Model file for the job. Use its own axes, mm. Face numbers are marked on the shaded views. A direction names the side the tool comes from. Round coordinates to 2 decimals unless told otherwise and drop trailing zeros. Loops run counter-clockwise (first coordinate to the right, second up) from the corner with the lowest first, then second, coordinate; pieces in that order, holes last. Notation, with made-up numbers: M -13,27.25 L 41,27.25 A33 cw 41,60.25 Z; hole C -31,49 d9. An arc over 180 degrees is marked long. Answer in a Markdown table with one row per item.
from build123d import *

# Parameters (mm, degrees)
F0_W     = 0.1
F0_H     = 20.0163984491
F0_W_2   = 0.2
F0_H_2   = 20
F0_W_3   = 0.3
F0_W_4   = 0.4
F0_W_5   = 0.5
F0_W_6   = 0.6
F0_W_7   = 0.7
F0_W_8   = 0.8
F0_W_9   = 0.9
F0_W_10  = 1
F0_R     = 0.05
F0_R_2   = 0.1
F0_R_3   = 0.15
F0_R_4   = 0.2
F0_R_5   = 0.25
F0_R_6   = 0.3
F0_R_7   = 0.35
F0_R_8   = 0.4
F0_R_9   = 0.45
F0_R_10  = 0.5
F1_DEPTH = 10
F2_W     = 1
F2_H     = 20
F2_W_2   = 0.2
F2_W_3   = 0.5
F2_W_4   = 0.9
F2_W_5   = 0.7
F2_W_6   = 0.8
F2_W_7   = 0.6
F2_R     = 0.35
F2_R_2   = 0.2
F2_R_3   = 0.15
F2_R_4   = 0.1
F2_W_8   = 0.3
F2_R_5   = 0.3
F2_R_6   = 0.4
F2_R_7   = 0.05
F2_R_8   = 0.45
F2_R_9   = 0.5
F2_R_10  = 0.25
F2_W_9   = 0.4
F2_W_10  = 0.1
F2_H_2   = 20.0163984491
F3_DEPTH = 50


with BuildPart() as f1:
    # F0 (on Top) → F1 (new body)
    with BuildSketch(Plane.XY):
        with BuildLine():
            Line((30, 29.7358127656), (-10, 29.7358127656))
            ThreePointArc((-10, 29.7358127656), (-24.1421356237, 23.8779483894), (-30, 9.7358127656))
            Line((-30, 9.7358127656), (-30, -22.3076807681))
            Line((-30, -22.3076807681), (10, -22.3076807681))
            ThreePointArc((10, -22.3076807681), (24.1421356237, -16.4498163918), (30, -2.3076807681))
            Line((30, -2.3076807681), (30, 29.7358127656))
        make_face()
        with Locations((-25.3179286689, -1.6637592667)):
            Rectangle(F0_W, F0_H, mode=Mode.SUBTRACT)
        with Locations((-20.1679286689, -1.6719584912)):
            Rectangle(F0_W_2, F0_H_2, mode=Mode.SUBTRACT)
        with Locations((-14.9179286689, -1.6719584912)):
            Rectangle(F0_W_3, F0_H_2, mode=Mode.SUBTRACT)
        with Locations((-9.5679286689, -1.6719584912)):
            Rectangle(F0_W_4, F0_H_2, mode=Mode.SUBTRACT)
        with Locations((-4.1179286689, -1.6719584912)):
            Rectangle(F0_W_5, F0_H_2, mode=Mode.SUBTRACT)
        with Locations((1.4320713311, -1.6719584912)):
            Rectangle(F0_W_6, F0_H_2, mode=Mode.SUBTRACT)
        with Locations((7.0820713311, -1.6719584912)):
            Rectangle(F0_W_7, F0_H_2, mode=Mode.SUBTRACT)
        with Locations((12.8320713311, -1.6719584912)):
            Rectangle(F0_W_8, F0_H_2, mode=Mode.SUBTRACT)
        with Locations((18.6820713311, -1.6719584912)):
            Rectangle(F0_W_9, F0_H_2, mode=Mode.SUBTRACT)
        with Locations((24.6320713311, -1.6719584912)):
            Rectangle(F0_W_10, F0_H_2, mode=Mode.SUBTRACT)
        with Locations((-25.3179286689, 13.3444399579)):
            Circle(F0_R, mode=Mode.SUBTRACT)
        with Locations((-20.1679286689, 13.3444399579)):
            Circle(F0_R_2, mode=Mode.SUBTRACT)
        with Locations((-14.9179286689, 13.3444399579)):
            Circle(F0_R_3, mode=Mode.SUBTRACT)
        with Locations((-9.5679286689, 13.3444399579)):
            Circle(F0_R_4, mode=Mode.SUBTRACT)
        with Locations((-4.1179286689, 13.3444399579)):
            Circle(F0_R_5, mode=Mode.SUBTRACT)
        with Locations((-25.2921710323, 18.3443736119)):
            Circle(F0_R, mode=Mode.SUBTRACT)
        with Locations((-20.1679286689, 18.3443736119)):
            Circle(F0_R_2, mode=Mode.SUBTRACT)
        with Locations((-14.9179286689, 18.3443736119)):
            Circle(F0_R_3, mode=Mode.SUBTRACT)
        with Locations((-9.5679286689, 18.3443736119)):
            Circle(F0_R_4, mode=Mode.SUBTRACT)
        with Locations((-4.1179286689, 18.3443736119)):
            Circle(F0_R_5, mode=Mode.SUBTRACT)
        with Locations((1.4320713311, 13.3444399579)):
            Circle(F0_R_6, mode=Mode.SUBTRACT)
        with Locations((7.0820713311, 13.3444399579)):
            Circle(F0_R_7, mode=Mode.SUBTRACT)
        with Locations((12.8320713311, 13.3444399579)):
            Circle(F0_R_8, mode=Mode.SUBTRACT)
        with Locations((18.6820713311, 13.3444399579)):
            Circle(F0_R_9, mode=Mode.SUBTRACT)
        with Locations((24.6320713311, 13.3444399579)):
            Circle(F0_R_10, mode=Mode.SUBTRACT)
        with Locations((1.4320713311, 18.3443736119)):
            Circle(F0_R_6, mode=Mode.SUBTRACT)
        with Locations((7.0820713311, 18.3443736119)):
            Circle(F0_R_7, mode=Mode.SUBTRACT)
        with Locations((12.8320713311, 18.3443736119)):
            Circle(F0_R_8, mode=Mode.SUBTRACT)
        with Locations((18.6820713311, 18.3443736119)):
            Circle(F0_R_9, mode=Mode.SUBTRACT)
        with Locations((24.6320713311, 18.3443736119)):
            Circle(F0_R_10, mode=Mode.SUBTRACT)
        with Locations((24.6320713311, -1.6719584912)):
            Rectangle(F0_W_10, F0_H_2)
        with Locations((18.6820713311, -1.6719584912)):
            Rectangle(F0_W_9, F0_H_2)
        with Locations((12.8320713311, -1.6719584912)):
            Rectangle(F0_W_8, F0_H_2)
        with Locations((7.0820713311, -1.6719584912)):
            Rectangle(F0_W_7, F0_H_2)
        with Locations((1.4320713311, -1.6719584912)):
            Rectangle(F0_W_6, F0_H_2)
        with Locations((-4.1179286689, -1.6719584912)):
            Rectangle(F0_W_5, F0_H_2)
        with Locations((-9.5679286689, -1.6719584912)):
            Rectangle(F0_W_4, F0_H_2)
        with Locations((-14.9179286689, -1.6719584912)):
            Rectangle(F0_W_3, F0_H_2)
        with Locations((-20.1679286689, -1.6719584912)):
            Rectangle(F0_W_2, F0_H_2)
        with Locations((-25.3179286689, -1.6637592667)):
            Rectangle(F0_W, F0_H)
        with Locations((24.6320713311, 13.3444399579)):
            Circle(F0_R_10)
        with Locations((18.6820713311, 13.3444399579)):
            Circle(F0_R_9)
        with Locations((12.8320713311, 13.3444399579)):
            Circle(F0_R_8)
        with Locations((7.0820713311, 13.3444399579)):
            Circle(F0_R_7)
        with Locations((1.4320713311, 13.3444399579)):
            Circle(F0_R_6)
        with Locations((-4.1179286689, 13.3444399579)):
            Circle(F0_R_5)
        with Locations((-9.5679286689, 13.3444399579)):
            Circle(F0_R_4)
        with Locations((-14.9179286689, 13.3444399579)):
            Circle(F0_R_3)
        with Locations((-20.1679286689, 13.3444399579)):
            Circle(F0_R_2)
        with Locations((-25.3179286689, 13.3444399579)):
            Circle(F0_R)
    extrude(amount=F1_DEPTH)

    # F2 (on face) → F3 (join)
    with BuildSketch(Plane.XY.offset(10)):
        with Locations((24.6320713311, -1.6719584912)):
            Rectangle(F2_W, F2_H)
        with Locations((-20.1679286689, -1.6719584912)):
            Rectangle(F2_W_2, F2_H)
        with Locations((-4.1179286689, -1.6719584912)):
            Rectangle(F2_W_3, F2_H)
        with Locations((18.6820713311, -1.6719584912)):
            Rectangle(F2_W_4, F2_H)
        with Locations((7.0820713311, -1.6719584912)):
            Rectangle(F2_W_5, F2_H)
        with Locations((12.8320713311, -1.6719584912)):
            Rectangle(F2_W_6, F2_H)
        with Locations((1.4320713311, -1.6719584912)):
            Rectangle(F2_W_7, F2_H)
        with Locations((7.0820713311, 13.3444399579)):
            Circle(F2_R)
        with Locations((-9.5679286689, 13.3444399579)):
            Circle(F2_R_2)
        with Locations((-14.9179286689, 13.3444399579)):
            Circle(F2_R_3)
        with Locations((-20.1679286689, 13.3444399579)):
            Circle(F2_R_4)
        with Locations((-14.9179286689, -1.6719584912)):
            Rectangle(F2_W_8, F2_H)
        with Locations((1.4320713311, 13.3444399579)):
            Circle(F2_R_5)
        with Locations((12.8320713311, 13.3444399579)):
            Circle(F2_R_6)
        with Locations((-25.3179286689, 13.3444399579)):
            Circle(F2_R_7)
        with Locations((18.6820713311, 13.3444399579)):
            Circle(F2_R_8)
        with Locations((24.6320713311, 13.3444399579)):
            Circle(F2_R_9)
        with Locations((-4.1179286689, 13.3444399579)):
            Circle(F2_R_10)
        with Locations((-9.5679286689, -1.6719584912)):
            Rectangle(F2_W_9, F2_H)
        with Locations((-25.3179286689, -1.6637592667)):
            Rectangle(F2_W_10, F2_H_2)
    extrude(amount=F3_DEPTH)


solid = f1.part
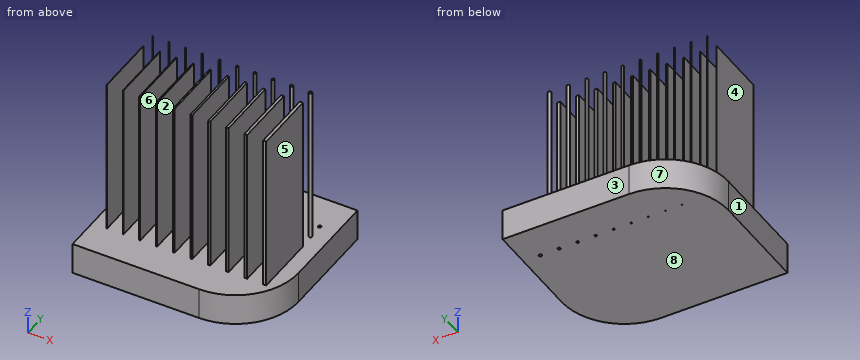
1. Saw through at A-A (z = 14). State how many separate pieces and enclosed holes the cut face has, and give its area (3 significant figures).
Verdict:
| item | result |
|---|---|
| separate pieces | 20 |
| enclosed holes | 0 |
| area | 113 mm² |
2. Tool access for the marked faces 4, 5, 6, 7 and 8: list every direction of +Z, -Z, +X, -X, +Y, -Y with a clear straight run to the whole face (end or side of a thin tool).
Verdict:
| item | result |
|---|---|
| face 4 | +Z, -X, +Y, -Y |
| face 5 | +Z, +X, +Y, -Y |
| face 6 | +Z, +Y, -Y |
| face 7 | +Z, -Z, -X, +Y |
| face 8 | -Z, +X, -X, +Y, -Y |
3. Wall check: probe 1 along Z at (x, y) = (-17, 9); probe 2 along Y at (x, z) = (-12, 9). Give the ranges that are in metal, low to high.
Verdict:
| item | result |
|---|---|
| probe 1 | z = 0 to 10 |
| probe 2 | y = -22.31 to 29.64 |
4. Saw through at C-C (x = -8). Write the cut outline in (y, z), and give its area (3 significant figures).
Verdict:
| item | result |
|---|---|
| outline | M -22.31,0 L 29.74,0 L 29.74,10 L -22.31,10 Z |
| area | 520 mm² |
5. Pin check, flat tips, straight feed: pin 1 (10 mm diameter, centred on x = 16.5, z = 50, fed in from -Y); pin 2 (12 mm diameter, centred on x = -22.5, z = 21, fed in from +Y); pin 3 (22 mm diameter, centred on y = 2.5, z = 43.5, fed in from -X); pin 4 (15.5 mm diameter, centred on x = -10, y = -1, fed in from +Z). Stop position of each tip, or through.
Verdict:
| item | result |
|---|---|
| pin 1 | stops at y = -11.67 |
| pin 2 | stops at y = 13.44 |
| pin 3 | stops at x = -25.37 |
| pin 4 | stops at z = 60 |
6. Mould opens along X. For the marked faces 1, 2 and 3 say: +X half, -X half, draft (parallel to the pull), parting line (faces both ways), or undercut.
Verdict:
| item | result |
|---|---|
| face 1 | -X half |
| face 2 | undercut |
| face 3 | draft |
7. Saw through at B-B (y = -17). Write the cut outline in (x, z).
Verdict:
| item | result |
|---|---|
| outline | M -30,0 L 23.57,0 L 23.57,10 L -30,10 Z |
